Can you work these out from the model? Positions are in its coordinate system, mm. A direction names the side the tool comes from. Coordinates: 2 decimals unless noted, no trailing zeros. Loops run counter-clockwise (first coordinate to the right, second up) from the corner with the lowest first, then second, coordinate; pieces in that order, holes last.
```python
from build123d import *

# Parameters (mm, degrees)
F1_DEPTH = 47.57
F2_R     = 8
F3_DEPTH = 25
F4_R     = 12.7
F5_DEPTH = 8.2
F6_R     = 2.5
F7_DEPTH = 50.801
F8_R     = 4
F9_DEPTH = 15.2


with BuildPart() as f1:
    # F0 (on Front) → F1 (new body, symmetric)
    with BuildSketch(Plane.XZ):
        Polygon((-25.4, 0), (0, 0), (25.4, 0), (25.4, 9.66), (17.44, 9.66), (17.44, 18), (0, 18), (-17.44, 18), (-17.44, 9.66), (-25.4, 9.66), align=None)
    extrude(amount=F1_DEPTH, both=True)

    # F2 (on face) → F3 (cut)
    with BuildSketch(Plane.XY.offset(18)):
        Circle(F2_R)
    extrude(amount=-F3_DEPTH, mode=Mode.SUBTRACT)

    # F4 (on face) → F5 (cut)
    with BuildSketch(Plane(origin=(0, 0, 0), x_dir=(1, 0, 0), z_dir=(0, 0, -1))):
        Circle(F4_R)
    extrude(amount=-F5_DEPTH, mode=Mode.SUBTRACT)

    # F6 (on face) → F7 (cut, through all)
    with BuildSketch(Plane(origin=(-25.4, 0, 0), x_dir=(0, -1, 0), z_dir=(-1, 0, 0))):
        with Locations((0, 4.2)):
            Circle(F6_R)
    extrude(amount=-F7_DEPTH, mode=Mode.SUBTRACT)

    # F8 (on face) → F9 (cut)
    with BuildSketch(Plane(origin=(0, 0, 0), x_dir=(1, 0, 0), z_dir=(0, 0, -1))):
        with Locations((0, -12.7)):
            Circle(F8_R)
    extrude(amount=-F9_DEPTH, mode=Mode.SUBTRACT)


solid = f1.part
```
Item 1: On a 3-axis mill with a long thin cutter (end or side, diameter ignored), from which of +Z, -Z, +X, -X, +Y, -Y can I reach the whole of each face in a straight line? I mean faces 1 (the face through (-17.44, -1, 14)), 2 (the face through (0, -9, 8.2)), 3 (the face through (17.44, -1, 14)). Say none if no direction works.
Results are:
face 1: +Z, -X, +Y, -Y
face 2: -Z
face 3: +Z, +X, +Y, -Y
Item 2: Suppose I cut it at B-B, the plane z = 16.25. Please give me the cut outline in (x, y).
Results are:
outline: (-17.44, -47.57) - (17.44, -47.57) - (17.44, 47.57) - (-17.44, 47.57) - close; hole circle Ø16 at (0, 0)
Item 3: Suppose I cut it at C-C, the plane z = 12.25. Please give me the cut outline in (x, y).
Results are:
outline: (-17.44, -47.57) - (17.44, -47.57) - (17.44, 47.57) - (-17.44, 47.57) - close; hole circle Ø16 at (0, 0); hole circle Ø8 at (0, 12.7)
Item 4: I need wall thicknesses on line 1 along Y through (x, z) = (0, 9.75); line 2 along Y through (x, z) = (0, 5); line 3 along Z through (x, y) = (22.75, 0). Which ranges of each line are inside material? Lowest first, please.
Results are:
line 1: y = -47.57 to -8, 8 to 8.7, 16.7 to 47.57
line 2: y = -47.57 to -12.7, 16.7 to 47.57
line 3: z = 0 to 1.7, 6.7 to 9.66
Item 5: Suppose I cut it at A-A, the plane x = 0. Please give me the cut outline in (y, z).
Results are:
outline: (-47.57, 0) - (-12.7, 0) - (-12.7, 8.2) - (-8, 8.2) - (-8, 18) - (-47.57, 18) - close; (8, 8.2) - (8.7, 8.2) - (8.7, 15.2) - (16.7, 15.2) - (16.7, 0) - (47.57, 0) - (47.57, 18) - (8, 18) - close
Item 6: Suppose I cut it at D-D, the plane y = -42. Please give me the cut outline in (x, z), plus the area to 3 significant figures.
Results are:
outline: (-25.4, 0) - (25.4, 0) - (25.4, 9.66) - (17.44, 9.66) - (17.44, 18) - (-17.44, 18) - (-17.44, 9.66) - (-25.4, 9.66) - close
area: 782 mm2
Item 7: We'd pull the mould along X, two halves only. Please class faces 4 (the face through (-21, -1, 9.66)), 5 (the face through (-25.4, -1, 7)), 6 (the face through (0, 13, 15.2)): +X half, -X half, draft (parallel to the pull), parting line (faces both ways), or undercut.
Results are:
face 4: draft
face 5: -X half
face 6: undercut
Item 8: I'm going to push flat-ended pins straight in: P1, Ø6.5, axis at x = -23, y = -6, coming from the +Z side; P2, Ø23, axis at x = 0, y = 0, coming from the -Z side; P3, Ø3, axis at y = 0, z = 4.2, coming from the +X side; P4, Ø4, axis at y = 21, z = 15, coming from the +X side. Where does each tip first touch, or does it pass through?
Results are:
P1: stops at z = 9.66
P2: stops at z = 8.2
P3: passes through
P4: stops at x = 17.44
